Solid Edge part; units mm, degrees
sketch "Sketch1" plane through (0, 0, 0) normal (0, -1, 0) x (1, 0, 0)
  line L0 (15, -25) -> (15, 25)
  line L1 (15, 25) -> (-15, 25)
  line L2 (-15, 25) -> (-15, -25)
  line L3 (-15, -25) -> (15, -25)
extrude "Protrusion1" add sketch "Sketch1" against normal blind 10
hole "Bohrung_1" at (0, 10, 10) direction (0, -1, 0) diameter 8 end through all counterbore diameter 9 counterbore depth 6
sketch "Sketch2" plane through (0, 10, 0) normal (0, 1, 0) x (1, 0, 0)
  line L0 (-15, 25) -> (15, 25)
  line L1 (15, 25) -> (15, -25)
  line L2 (15, -25) -> (-15, -25)
  line L3 (-15, -25) -> (-15, 25)
  circle A0 centre (0, -10) radius 14.75
extrude "Extrusionsausprägung_2" cut sketch "Sketch2" against normal blind 1.3
fillet "Verrundung_1" radius 1 4 edges at (-15, 4.35, 25) (15, 4.35, 25) (15, 4.35, -25) (-15, 4.35, -25)
hole "Bohrung_2" at (-12, 10, 10) direction (0, -1, 0) diameter 2.459 end through all
hole "Hole1" at (12, 10, 10) direction (0, -1, 0) diameter 2.459 end through all
hole "Bohrung_4" at (10.48, 0, -5.75) direction (0, 1, 0) diameter 2.459 depth 15 thread major 3 thread length 10
hole "Hole2" at (-10.48, 0, -5.75) direction (0, 1, 0) diameter 2.459 depth 15 thread major 3 thread length 10
Can you work these out from the model? Positions are in its coordinate system, mm. A direction names the side the tool comes from. Give positions to 0.01 mm unless a question says otherwise; leave off trailing zeros. Order: outer loops, then holes, each group sorted by start corner. A loop starts at its lowest first (then second) coordinate and runs counter-clockwise, first axis right, second up. Notation, with made-up numbers: (-10.75, 76) - (33.25, 76) arc R26 ccw to (33.25, 111) - close; hole circle Ø8 at (-8.75, 86.25). An arc over 180 degrees is marked (long way). Use a Markdown table: item, result. Add a question column.
Q1. If we section it at C-C on z = 10: Write out the boundary of the cut face in (x, y), plus the area to 3 significant figures.
Q2. Please list where these lines run through material, in increasing order: line 1 along X through (y, z) = (7, -5.75); line 2 along X through (y, z) = (6, 10); line 3 along X through (y, z) = (3.5, 10).
Q3. I'm going to push a flat-ended pin straight in: pin 1 (4 mm diameter, centred on x = 11, z = -4.5, fed in from -Y). Where does the tip first touch, or does it pass through?
Q4. If we section it at D-D on x = -3: Write out the boundary of the cut face in (y, z), plus the area to 3 significant figures.
Q5. If we section it at A-A on y = 2.5: Write out the boundary of the cut face in (x, z), plus the area to 3 significant figures.
Q6. If we section it at B-B on z = -5.75: Write out the boundary of the cut face in (x, y).
Q7. If we mould it in two halves opening along X, with no side actions, what happens to faces 1 (the flat face through (3.5, 10, 6.9)), 2 (the cylindrical face through (-14.699, 4.411, -24.715)), 3 (the cylindrical face through (11.228, 4.411, -4.774)), 4 (the cylindrical face through (14.699, 4.411, 24.715))? For each: released by +X, released by -X, zero draft, split by the parting line, or undercut.
Q8. On a 3-axis mill with a long thin cutter (end or side, diameter ignored), from which of +Z, -Z, +X, -X, +Y, -Y can I reach the whole of each face in a straight line? I mean faces 5 (the cylindrical face through (-11.631, 5.07, 11.173)), 6 (the cylindrical face through (-1.352, 6.958, 14.292)). Say none if no direction works.
Answers follow:
| question | item | result |
|---|---|---|
| 1 | outline | (-15, 0) - (-13.23, 0) - (-13.23, 10) - (-14.75, 10) - (-14.75, 8.7) - (-15, 8.7) - close; (-10.77, 0) - (-4, 0) - (-4, 4) - (-4.5, 4) - (-4.5, 10) - (-10.77, 10) - close; (4, 0) - (10.77, 0) - (10.77, 10) - (4.5, 10) - (4.5, 4) - (4, 4) - close; (13.23, 0) - (15, 0) - (15, 8.7) - (14.75, 8.7) - (14.75, 10) - (13.23, 10) - close |
| 1 | area | 164 mm^2 |
| 2 | line 1 | x = -15 to -11.71, -9.25 to 9.25, 11.71 to 15 |
| 2 | line 2 | x = -15 to -13.23, -10.77 to -4.5, 4.5 to 10.77, 13.23 to 15 |
| 2 | line 3 | x = -15 to -13.23, -10.77 to -4, 4 to 10.77, 13.23 to 15 |
| 3 | pin 1 | stops at y = 0 |
| 4 | outline | (0, -25) - (8.7, -25) - (8.7, -4.44) - (10, -4.44) - (10, 6.65) - (4, 6.65) - (4, 7.35) - (0, 7.35) - close; (0, 12.65) - (4, 12.65) - (4, 13.35) - (10, 13.35) - (10, 24.44) - (8.7, 24.44) - (8.7, 25) - (0, 25) - close |
| 4 | area | 411 mm^2 |
| 5 | outline | (-15, -24) arc R1 ccw to (-14, -25) - (14, -25) arc R1 ccw to (15, -24) - (15, 24) arc R1 ccw to (14, 25) - (-14, 25) arc R1 ccw to (-15, 24) - close; hole circle Ø2.46 at (-12, 10); hole circle Ø2.46 at (-10.48, -5.75); hole circle Ø8 at (0, 10); hole circle Ø2.46 at (10.48, -5.75); hole circle Ø2.46 at (12, 10) |
| 5 | area | 1,430 mm^2 |
| 6 | outline | (-15, 0) - (-11.71, 0) - (-11.71, 8.7) - (-15, 8.7) - close; (-9.25, 0) - (9.25, 0) - (9.25, 8.7) - (-9.25, 8.7) - close; (11.71, 0) - (15, 0) - (15, 8.7) - (11.71, 8.7) - close |
| 7 | face 1 | zero draft |
| 7 | face 2 | released by -X |
| 7 | face 3 | undercut |
| 7 | face 4 | released by +X |
| 8 | face 5 | +Y, -Y |
| 8 | face 6 | +Y |
